Build history of the part. All positions in model axes, mm. A direction names the side the tool comes from. Give positions to 0.01 mm unless a question says otherwise; leave off trailing zeros. Order: outer loops, then holes, each group sorted by start corner. A loop starts at its lowest first (then second) coordinate and runs counter-clockwise, first axis right, second up. Notation, with made-up numbers: (-17, -25.75) - (2, -25.75) arc R33 ccw to (2, 11.25) - close; hole circle Ø7 at (5.25, 77.5). An arc over 180 degrees is marked (long way). Write each question's results on one line, items separated by ' | '. Start each with the question number.
1) Cut at D-D on x = 3. List the corners of the cut face in (y, z).
2) Cut at C-C on z = 2. List the corners of the cut face in (x, y), plus the area to 3 significant figures.
3) Tool access for faces 1 (the face through (0.164, -10.69, 5.543)), 2 (the face through (-4.4, -2, 0)), 3 (the face through (4.4, -2, 0)): list every direction of +Z, -Z, +X, -X, +Y, -Y with a clear straight run to the whole face (end or side of a thin tool).
4) Cut at A-A on x = 0. List the corners of the cut face in (y, z).
5) Drop flat-ended pins along their axis: pin 1 Ø7 at (x, y) = (-1, 1) entering from +Z; pin 2 Ø5 at (x, y) = (-3, -8.5) entering from +Z; pin 3 Ø1.5 at (y, z) = (1, 0.5) entering from +X; pin 4 Ø1.5 at (x, y) = (-5, -2) entering from -Z. Give the stop position or say it passes through.
6) Drill centre lines: line 1 along Y through (x, z) = (0, -1.95); line 2 along Y through (x, z) = (-4.25, 5.5); line 3 along Z through (x, y) = (-2, 0). Where is each one in solid material? Low to high. Write a range as from..to.
7) Cut at B-B on y = 3.5. List the corners of the cut face in (x, z).
from build123d import *

# Parameters (mm, degrees)
F0_W          = 8.8
F0_H          = 20
F0_R          = 2
F1_DEPTH      = 2.8
F1_DEPTH_BACK = 2.8
F2_W          = 8.8
F2_H          = 5.6
F3_DEPTH      = 1.4
F4_START      = 1.4
F4_DEPTH      = 2
F5_R          = 3.7903152929


with BuildPart() as f1:
    # F0 (on Top) → F1 (new body, two sides)
    with BuildSketch(Plane.XY) as f1_sk:
        Rectangle(F0_W, F0_H)
        with Locations((0, 4.8)):
            Circle(F0_R, mode=Mode.SUBTRACT)
    extrude(amount=F1_DEPTH)
    extrude(f1_sk.sketch, amount=-F1_DEPTH_BACK)

    # F2 (on face) → F3 (join)
    with BuildSketch(Plane.XZ.offset(10)):
        with BuildLine():
            Line((4.4, -2.8), (5.2114805567, -2.8))
            ThreePointArc((5.2114805567, -2.8), (0, 5.5456768073), (-5.2114805567, -2.8))
            Line((-5.2114805567, -2.8), (-4.4, -2.8))
            Line((-4.4, -2.8), (-4.4, 2.8))
            Line((-4.4, 2.8), (4.4, 2.8))
            Line((4.4, 2.8), (4.4, -2.8))
        make_face()
        Rectangle(F2_W, F2_H)
    extrude(amount=F3_DEPTH)

    # F2 (on face) → F4 (join)
    with BuildSketch(Plane.XZ.offset(10).offset(F4_START)):
        Rectangle(F2_W, F2_H)
        with BuildLine():
            Line((4.4, -2.8), (5.2114805567, -2.8))
            ThreePointArc((5.2114805567, -2.8), (0, 5.5456768073), (-5.2114805567, -2.8))
            Line((-5.2114805567, -2.8), (-4.4, -2.8))
            Line((-4.4, -2.8), (-4.4, 2.8))
            Line((-4.4, 2.8), (4.4, 2.8))
            Line((4.4, 2.8), (4.4, -2.8))
        make_face()
        with BuildLine():
            ThreePointArc((-5.2114805567, -2.8), (0, 5.5456768073), (5.2114805567, -2.8))
            Line((5.2114805567, -2.8), (9.1525695623, -2.8))
            ThreePointArc((9.1525695623, -2.8), (0, 9.2456768073), (-9.1525695623, -2.8))
            Line((-9.1525695623, -2.8), (-5.2114805567, -2.8))
        make_face()
    extrude(amount=F4_DEPTH)

    # F5
    f5_edges = [f1.edges().sort_by_distance(p)[0] for p in [
        (4.4, 10, 0),
        (-4.4, 10, 0),
    ]]
    fillet(f5_edges, radius=F5_R)


solid = f1.part
Results:
1) outline: (-13.4, -2.8) - (9.15, -2.8) - (9.15, 2.8) - (-10, 2.8) - (-10, 4.71) - (-11.4, 4.71) - (-11.4, 8.76) - (-13.4, 8.76) - close
2) outline: (-9.23, -13.4) - (9.23, -13.4) - (9.23, -11.4) - (5.34, -11.4) - (5.34, -10) - (4.4, -10) - (4.4, 6.21) arc R3.79 ccw to (0.61, 10) - (-0.61, 10) arc R3.79 ccw to (-4.4, 6.21) - (-4.4, -10) - (-5.34, -10) - (-5.34, -11.4) - (-9.23, -11.4) - close; hole circle Ø4 at (0, 4.8) | area: 209 mm^2
3) face 1: +Y | face 2: +Z, -Z, -X, +Y | face 3: +Z, -Z, +X, +Y
4) outline: (-13.4, -2.8) - (2.8, -2.8) - (2.8, 2.8) - (-10, 2.8) - (-10, 5.55) - (-11.4, 5.55) - (-11.4, 9.25) - (-13.4, 9.25) - close; (6.8, -2.8) - (10, -2.8) - (10, 2.8) - (6.8, 2.8) - close
5) pin 1: z = 2.8 | pin 2: z = 5.46 | pin 3: x = 4.4 | pin 4: z = -2.8
6) line 1: -13.4..2.8, 6.8..10 | line 2: -13.4..-11.4 | line 3: -2.8..2.8
7) outline: (-4.4, -2.8) - (-1.52, -2.8) - (-1.52, 2.8) - (-4.4, 2.8) - close; (1.52, -2.8) - (4.4, -2.8) - (4.4, 2.8) - (1.52, 2.8) - close
